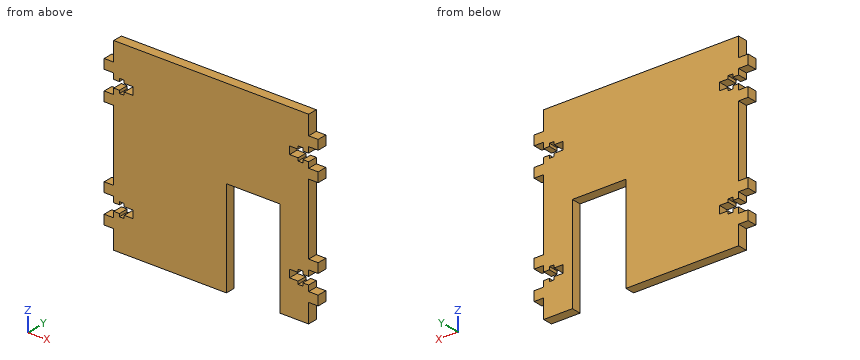
from build123d import *

# Parameters (mm, degrees)
BOSS_EXTRUDE2_DEPTH = 5


with BuildPart() as part:
    # Sketch2 → Boss-Extrude2 (new body)
    with BuildSketch(Plane(origin=(0, 0, 0), x_dir=(1, 0, 0), z_dir=(0, 1, 0))):
        Polygon((143.481880544, 36.328109734), (143.481880544, 33.328109734), (140.481880544, 33.328109734), (140.481880544, 34.828109734), (137.981880544, 34.828109734), (137.981880544, 33.328109734), (133.481880544, 33.328109734), (133.481880544, 29.328109734), (137.981880544, 29.328109734), (137.981880544, 27.828109734), (140.481880544, 27.828109734), (140.481880544, 29.328109734), (143.481880544, 29.328109734), (143.481880544, 26.328109734), (148.481880544, 26.328109734), (148.481880544, 21.328109734), (143.481880544, 21.328109734), (143.481880544, -15.671890266), (148.481880544, -15.671890266), (148.481880544, -20.671890266), (143.481880544, -20.671890266), (143.481880544, -23.671890266), (140.481880544, -23.671890266), (140.481880544, -22.171890266), (137.981880544, -22.171890266), (137.981880544, -23.671890266), (133.481880544, -23.671890266), (133.481880544, -27.671890266), (137.981880544, -27.671890266), (137.981880544, -29.171890266), (140.481880544, -29.171890266), (140.481880544, -27.671890266), (143.481880544, -27.671890266), (143.481880544, -30.671890266), (148.481880544, -30.671890266), (148.481880544, -35.671890266), (143.481880544, -35.671890266), (143.481880544, -45.671890266), (41.481880544, -45.671890266), (41.481880544, -35.671890266), (36.481880544, -35.671890266), (36.481880544, -30.671890266), (41.481880544, -30.671890266), (41.481880544, -27.671890266), (44.481880544, -27.671890266), (44.481880544, -29.171890266), (46.981880544, -29.171890266), (46.981880544, -27.671890266), (51.481880544, -27.671890266), (51.481880544, -23.671890266), (46.981880544, -23.671890266), (46.981880544, -22.171890266), (44.481880544, -22.171890266), (44.481880544, -23.671890266), (41.481880544, -23.671890266), (41.481880544, -20.671890266), (36.481880544, -20.671890266), (36.481880544, -15.671890266), (41.481880544, -15.671890266), (41.481880544, 21.328109734), (36.481880544, 21.328109734), (36.481880544, 26.328109734), (41.481880544, 26.328109734), (41.481880544, 29.328109734), (44.481880544, 29.328109734), (44.481880544, 27.828109734), (46.981880544, 27.828109734), (46.981880544, 29.328109734), (51.481880544, 29.328109734), (51.481880544, 33.328109734), (46.981880544, 33.328109734), (46.981880544, 34.828109734), (44.481880544, 34.828109734), (44.481880544, 33.328109734), (41.481880544, 33.328109734), (41.481880544, 36.328109734), (36.481880544, 36.328109734), (36.481880544, 41.328109734), (41.481880544, 41.328109734), (41.481880544, 51.328109734), (100.481880544, 51.328109734), (100.481880544, 0.828109734), (128.481880544, 0.828109734), (128.481880544, 51.328109734), (143.481880544, 51.328109734), (143.481880544, 41.328109734), (148.481880544, 41.328109734), (148.481880544, 36.328109734), align=None)
    extrude(amount=BOSS_EXTRUDE2_DEPTH)


solid = part.part
CAD build for the part. Positions are in the model's coordinates, mm. Round coordinates to 2 decimals unless told otherwise and drop trailing zeros. Order: outer loops, then holes, each group sorted by start corner. A loop starts at its lowest first (then second) coordinate and runs counter-clockwise, first axis right, second up. Notation, with made-up numbers: M 30.5,10.5 L 58.5,10.5 A15 cw 58.5,28.5 Z; hole C 74,79.5 d5. An arc over 180 degrees is marked long. Use one line per item in the form item = value.
Q1. Saw through at A-A on z = 37. Give the cut face in (x, y), then the cut area to 3 significant figures.
Recorded:
outline = M 41.48,0 L 143.48,0 L 143.48,5 L 41.48,5 Z
area = 510 mm^2
Q2. Probe L1, parallel to X at y = 2.3, z = 23.5; L2, parallel to Z at x = 144, y = 1.75; L3, parallel to Z at x = 135, y = 2.15. List the from-to ranges inside material, lowest first.
Recorded:
L1 = 41.48 to 44.48, 46.98 to 137.98, 140.48 to 143.48
L2 = -41.33 to -36.33, -26.33 to -21.33, 15.67 to 20.67, 30.67 to 35.67
L3 = -51.33 to -33.33, -29.33 to 23.67, 27.67 to 45.67
Q3. Saw through at B-B on x = 112.5. Give the cut face in (y, z), then the cut area to 4 significant figures.
Recorded:
outline = M 0,-0.83 L 5,-0.83 L 5,45.67 L 0,45.67 Z
area = 232.5 mm^2
Q4. Flat gauge pins, fed straight in: P1, Ø1.2, axis at y = 2, z = 28.5, coming from the -X side; P2, Ø3, axis at y = 0.5, z = -11, coming from the +X side; P3, Ø1.5, axis at x = 146.5, y = 2.5, coming from the -Z side. Where does each tip first touch, or does it go through?
Recorded:
P1 = 41.48
P2 = 143.48
P3 = -41.33
